Here's how the part is built. I have some questions about the finished solid (model axes, mm). Coordinates: 2 decimals unless noted, no trailing zeros. Write each loop counter-clockwise with the first axis right and the second up, starting at its lowest first coordinate (ties: lowest second). Pieces come first, ordered by that corner, then holes. Notation, with made-up numbers: (41.25, 40.25) -> (90.25, 40.25) arc R34 ccw to (90.25, 72.25) -> close; hole circle Ø8 at (11, 29). An arc over 180 degrees is marked (long way). Use a Markdown table: item, result. Add a question column.
Item 1: If I drill on line 1 along X through (y, z) = (49.25, 70); line 2 along Z through (x, y) = (-71, 45.5); line 3 along Z through (x, y) = (-55, 47.75), over which ranges is the centre line in solid material (lowest first)? Write a range as from..to.
Item 2: Imagine slicing it at C-C, the plane x = -106. Write out the boundary of the cut face in (y, z).
Item 3: Imagine slicing it at A-A, the plane y = 43.5. Write out the boundary of the cut face in (x, z), and give its area (3 significant figures).
Item 4: Will these pins go through, and if not, where does the flat tip stop? pin 1 Ø1.5 at (x, y) = (-44, 42) entering from -Z; pin 2 Ø5 at (y, z) = (43.5, 30.5) entering from -X; pin 3 Ø2 at (y, z) = (46, 17) entering from +X.
Item 5: Imagine slicing it at B-B, the plane z = 38. Write out the boundary of the cut face in (x, y), and give its area (3 significant figures).
Solid Edge part; units mm, degrees
sketch "Sketch1" plane through (0, 0, 0) normal (0, 0, 1) x (1, 0, 0)
  line L0 (-85.0132, 40.6343) -> (-75.0132, 40.6343)
  line L1 (-75.0132, 40.6343) -> (-75.0132, 50.6343)
  line L2 (-75.0132, 50.6343) -> (-85.0132, 50.6343)
  line L3 (-85.0132, 50.6343) -> (-85.0132, 40.6343)
  dimension "D1" = 75.0132
  dimension "D2" = 75.0132
extrude "Protrusion1" add sketch "Sketch1" along normal blind 100
sketch "Sketch2" plane through (-30.0132, 45.6343, 50) normal (1, 0, 0) x (0, 0, -1)
  circle A0 centre (-53, 0) radius 5
extrude "ExtrudedProtrusion_2" add sketch "Sketch2" against normal blind 100
Ans:
| question | item | result |
|---|---|---|
| 1 | line 1 | x = -85.01..-75.01 |
| 1 | line 2 | z = 98..108 |
| 1 | line 3 | z = 98.47..107.53 |
| 2 | outline | circle Ø10 at (45.63, 103) |
| 3 | outline | (-130.01, 98.48) -> (-85.01, 98.48) -> (-85.01, 0) -> (-75.01, 0) -> (-75.01, 98.48) -> (-30.01, 98.48) -> (-30.01, 107.52) -> (-130.01, 107.52) -> close |
| 3 | area | 1,890 mm^2 |
| 4 | pin 1 | stops at z = 98.92 |
| 4 | pin 2 | stops at x = -85.01 |
| 4 | pin 3 | stops at x = -75.01 |
| 5 | outline | (-85.01, 40.63) -> (-75.01, 40.63) -> (-75.01, 50.63) -> (-85.01, 50.63) -> close |
| 5 | area | 100 mm^2 |
